from build123d import *

# Parameters (mm, degrees)
CUT_EXTRUDE_1_DEPTH = 1
FILLET_1_R          = 0.1


with BuildPart() as part:
    # 草图1 → 旋转2 (revolve)
    with BuildSketch(Plane(origin=(0, 0, 0), x_dir=(0, 0, -1), z_dir=(1, 0, 0))):
        with BuildLine():
            Line((0, 2.250343623), (0, 1))
            Line((0, 1), (0, 0))
            Line((0, 0), (1, 0))
            Line((1, 0), (1, 1))
            Line((1, 1), (1.248177586, 0))
            Line((1.248177586, 0), (51.5, 0))
            Line((51.5, 0), (51.5, 1.5))
            Line((51.5, 1.5), (1.5, 1.5))
            Line((1.5, 1.5), (1.5, 2.8))
            ThreePointArc((1.5, 2.8), (0.701231865, 2.658258964), (0, 2.250343623))
        make_face()
    revolve(axis=Axis((0, 0, 0), (0, 0, -1)))

    # 草图2 → 切除-拉伸1 (cut)
    with BuildSketch(Plane.XY):
        Polygon((0, 1.154700538), (-1, 0.577350269), (-1, -0.577350269), (0, -1.154700538), (1, -0.577350269), (1, 0.577350269), align=None)
    extrude(amount=-CUT_EXTRUDE_1_DEPTH, mode=Mode.SUBTRACT)

    # 圆角1
    fillet_1_edges = [part.edges().sort_by_distance(p)[0] for p in [
        (0, -1.5, -51.5),
    ]]
    fillet(fillet_1_edges, radius=FILLET_1_R)


solid = part.part
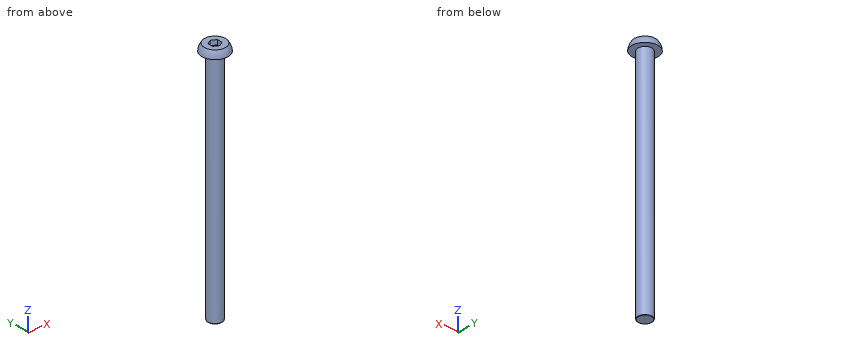
Work out the finished part from the listing and answer in its coordinate system (mm). Give positions to 0.01 mm unless a question says otherwise; leave off trailing zeros. Loops run counter-clockwise (first coordinate to the right, second up) from the corner with the lowest first, then second, coordinate; pieces in that order, holes last. Notation, with made-up numbers: M -32,47.5 L -5,47.5 A19 ccw -5,78.5 Z; hole C 31,18.25 d3. An arc over 180 degrees is marked long. Use CSV: the item, a comma, the result in double quotes.
1) Given P1, Ø3, axis at x = 2, z = -30, coming from the +Y side; P2, Ø1, axis at x = 0.5, y = -2, coming from the -Z side; P3, Ø1.5, axis at y = 0.5, z = -40, coming from the -X side, each flat-ended and moving along its own axis, determine where each tip first touches the part or whether it passes through.
Answer:
P1,"y = 1.41"
P2,"z = -1.5"
P3,"x = -1.5"
2) Find section A-A on z = -15. Write down the section's boundary in (x, y).
Answer:
outline,"C 0,0 d3"
3) Consider L1, parallel to X at y = 0, z = -15; L2, parallel to Y at x = 0.15, z = -17; L3, parallel to Z at x = -1.1, y = 1.4. Determine where each line is inside the solid, lowest interval first.
Answer:
L1,"-1.5 to 1.5"
L2,"-1.49 to 1.49"
L3,"-1.5 to 0"
